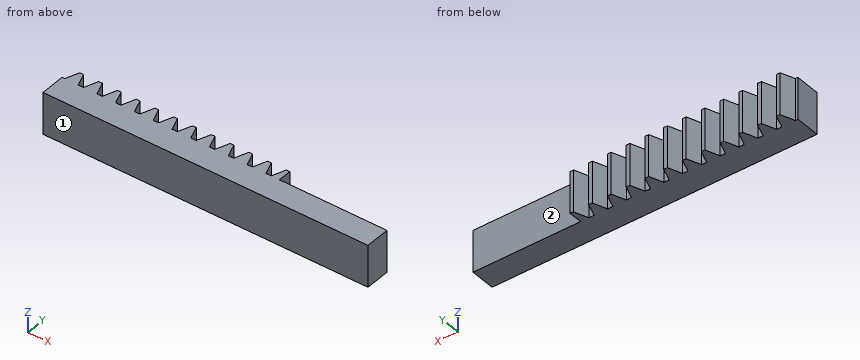
```python
from build123d import *

# Parameters (mm, degrees)
BLANKSKE_W         = 21.75
BLANKSKE_H         = 2.55
BLANK_DEPTH        = 2.8
TOOTHCUTSIM_DEPTH  = 23.077250735
TEETHCUTS_COUNT    = 18
TEETHCUTS_PITCH    = 1.25663706
SKETCH1_W          = 7.2
SKETCH1_H          = 0.9
CUT_EXTRUDE1_DEPTH = 23.077250735


with BuildPart() as part:
    # BlankSke → Blank (new body)
    with BuildSketch(Plane.XY):
        with Locations((10.875, 1.275)):
            Rectangle(BLANKSKE_W, BLANKSKE_H)
    extrude(amount=-BLANK_DEPTH)

    # TooCutSkeSim → ToothCutSim (cut, through all)
    with BuildSketch(Plane.XY):
        Polygon((0.177174148, 1.65), (-0.177174148, 1.65), (-0.513992203, 2.5754), (0.513992203, 2.5754), align=None)
    toothcutsim = extrude(amount=-TOOTHCUTSIM_DEPTH, mode=Mode.SUBTRACT)

    # TeethCuts: ToothCutSim ×18
    with Locations(*[(i * TEETHCUTS_PITCH, 0, 0) for i in range(1, TEETHCUTS_COUNT)]):
        add(toothcutsim, mode=Mode.SUBTRACT)

    # Sketch1 → Cut-Extrude1 (cut, through all)
    with BuildSketch(Plane.XY):
        with Locations((18.15, 2.1)):
            Rectangle(SKETCH1_W, SKETCH1_H)
    extrude(amount=-CUT_EXTRUDE1_DEPTH, mode=Mode.SUBTRACT)


solid = part.part
```
Geometry: final body of the model. Coordinates: model frame, mm. Face numbers are marked on the shaded views. A direction names the side the tool comes from. Give positions to 0.01 mm unless a question says otherwise; leave off trailing zeros. Loops run counter-clockwise (first coordinate to the right, second up) from the corner with the lowest first, then second, coordinate; pieces in that order, holes last. Notation, with made-up numbers: (57, 55.5) -> (106, 55.5) arc R17 ccw to (106, 70.5) -> close; hole circle Ø3 at (85.5, -17.5). An arc over 180 degrees is marked (long way). Use one line per item in the form item = value.
Item 1: Section query B-B on y = 2.3. Give the number of separate pieces and of enclosed holes in the cut face, and give its area (3 significant figures).
A:
separate_pieces = 12
enclosed_holes = 0
area = 14.1 mm^2
Item 2: Line query: probe 1 along Y at (x, z) = (14.75, -2.45). Output: solid intervals per line, ascending.
A:
probe_1 = 0 to 1.65
Item 3: Section query A-A on x = 17.75. Output: boundary loops of the cut face in (y, z).
A:
outline = (0, -2.8) -> (1.65, -2.8) -> (1.65, 0) -> (0, 0) -> close
Item 4: Access query for the marked faces 1 and 2. Directions: +Z, -Z, +X, -X, +Y, -Y. A direction counts if a zero-diameter tool reaches every point of the face in a straight line with its end or side. Return the directions, or none.
A:
face_1 = +Z, -Z, +X, -X, -Y
face_2 = +Z, -Z, +X, +Y
Item 5: Pin query (flat end, axial travel): P1, Ø0.8, axis at x = 17.5, z = -1, coming from the +Y side; P2, Ø1, axis at y = 1, z = -1.5, coming from the -X side. Return the tip coordinate at first contact, or that it passes through.
A:
P1 = 1.65
P2 = 0
